from build123d import *
from build123d import SkipClean  # not in build123d's __all__

# Parameters (mm, degrees)
F0_R     = 0.75
F0_R_2   = 2
F1_DEPTH = 1.8
F2_R     = 2
F3_DEPTH = 1.5


with BuildPart() as f1:
    # F0 (on Top) → F1 (new body)
    with BuildSketch(Plane.XY):
        with BuildLine():
            Line((-14.1428571429, -1.9948914348), (-0.2142857143, -2.9923371522))
            ThreePointArc((-0.2142857143, -2.9923371522), (3, 0), (-0.2142857143, 2.9923371522))
            Line((-0.2142857143, 2.9923371522), (-14.1428571429, 1.9948914348))
            ThreePointArc((-14.1428571429, 1.9948914348), (-16, 0), (-14.1428571429, -1.9948914348))
        make_face()
        with Locations((-14.5, 0)):
            Circle(F0_R, mode=Mode.SUBTRACT)
        with Locations((-12.5, 0)):
            Circle(F0_R, mode=Mode.SUBTRACT)
        with Locations((-10.5, 0)):
            Circle(F0_R, mode=Mode.SUBTRACT)
        Circle(F0_R_2, mode=Mode.SUBTRACT)
    extrude(amount=F1_DEPTH)

    # F2 (on face) → F3 (join)
    with BuildSketch(Plane(origin=(0, 0, 0), x_dir=(1, 0, 0), z_dir=(0, 0, -1))):
        with BuildLine():
            ThreePointArc((-0.2142857143, -2.9923371522), (3, 0), (-0.2142857143, 2.9923371522))
            ThreePointArc((-0.2142857143, 2.9923371522), (-3, 0), (-0.2142857143, -2.9923371522))
        make_face()
        Circle(F2_R, mode=Mode.SUBTRACT)
    with SkipClean():  # cleaning this boolean's faces spoils the solid; the shape is the same uncleaned
        extrude(amount=F3_DEPTH)


solid = f1.part
Model file for the job. Use its own axes, mm. Round coordinates to 2 decimals unless told otherwise and drop trailing zeros. Order: outer loops, then holes, each group sorted by start corner. A loop starts at its lowest first (then second) coordinate and runs counter-clockwise, first axis right, second up.
(1) Band-saw the part on B-B (y = 0). List the corners of the cut face in (x, z), then the cut area to 3 significant figures.
(2) Pin check, flat tips, straight feed: pin 1 (1 mm diameter, centred on x = -12, z = 0.5, fed in from -Y); pin 2 (3 mm diameter, centred on x = -5.5, y = -0.5, fed in from -Z). Stop position of each tip, or through.
(3) Band-saw the part on A-A (x = 0). List the corners of the cut face in (y, z).
(4) Band-saw the part on D-D (z = -0.45). List the corners of the cut face in (x, y).
(5) Band-saw the part on C-C (z = 1.3). List the corners of the cut face in (x, y).
(6) Drill centre lines: line 1 (Y direction, x = 0, z = 1.1); line 2 (Z direction, x = -6.5, y = -2.4); line 3 (X direction, y = -0.35, z = -0.4). Where is each one in solid material? Low to high.
(7) Pull direction Y, two halves, no side cores. Call faces 1 (the face through (-13.25, 0.03, 0.89)), 2 (the face through (-7.1, 2.5, 0.9)), 3 (the face through (-16, 0, 1)): released by +Y, released by -Y, zero draft, split by the parting line, or undercut.
Verdict:
1. outline: (-16, 0) - (-15.25, 0) - (-15.25, 1.8) - (-16, 1.8) - close; (-13.75, 0) - (-13.25, 0) - (-13.25, 1.8) - (-13.75, 1.8) - close; (-11.75, 0) - (-11.25, 0) - (-11.25, 1.8) - (-11.75, 1.8) - close; (-9.75, 0) - (-3, 0) - (-3, -1.5) - (-2, -1.5) - (-2, 1.8) - (-9.75, 1.8) - close; (2, -1.5) - (3, -1.5) - (3, 1.8) - (2, 1.8) - close
1. area: 21.9 mm2
2. pin 1: stops at y = -2.18
2. pin 2: stops at z = 0
3. outline: (-3, -1.5) - (-2, -1.5) - (-2, 1.8) - (-3, 1.8) - close; (2, -1.5) - (3, -1.5) - (3, 1.8) - (2, 1.8) - close
4. outline: circle Ø6 at (0, 0); hole circle Ø4 at (0, 0)
5. outline: (-14.14, -1.99) - (-0.21, -2.99) arc R3 ccw (long way) to (-0.21, 2.99) - (-14.14, 1.99) arc R2 ccw to start; hole circle Ø1.5 at (-14.5, 0); hole circle Ø1.5 at (-12.5, 0); hole circle Ø1.5 at (-10.5, 0); hole circle Ø4 at (0, 0)
6. line 1: y = -3 to -2, 2 to 3
6. line 2: z = 0 to 1.8
6. line 3: x = -2.98 to -1.97, 1.97 to 2.98
7. face 1: undercut
7. face 2: released by +Y
7. face 3: split by the parting line
